```python
from build123d import *
from OCP.BRepFilletAPI import BRepFilletAPI_MakeChamfer

# Parameters (mm, degrees)
SKETCH_1_W               = 70
SKETCH_1_H               = 60
EXTRUDE_1_DEPTH          = 15
SKETCH_2_R               = 11.5
EXTRUDE_3_DEPTH          = 5
CUT_EXTRUDE_1_DEPTH      = 69.745908969
CUT_EXTRUDE_1_DEPTH_BACK = 69.745908969
SKETCH_3_W               = 50
SKETCH_3_H               = 5
CHAMFER_1_SIZE           = 1.2
CHAMFER_1_SIZE2          = 0.692820323
CHAMFER_2_SIZE           = 1.2
CHAMFER_2_SIZE_2         = 0.692820323
CHAMFER_3_SIZE           = 1.2
CHAMFER_3_SIZE_2         = 0.692820323
CHAMFER_4_SIZE           = 1.2
CHAMFER_4_SIZE2          = 0.692820323


with BuildPart() as part:
    # 스케치1 → 보스-돌출1 (new body)
    with BuildSketch(Plane(origin=(0, 0, 0), x_dir=(1, 0, 0), z_dir=(0, 1, 0))):
        Rectangle(SKETCH_1_W, SKETCH_1_H)
    extrude(amount=EXTRUDE_1_DEPTH)

    # 스케치2 → 보스-돌출3 (add, symmetric)
    with BuildSketch(Plane(origin=(0, 0, 0), x_dir=(0, 0, -1), z_dir=(1, 0, 0))):
        with BuildLine():
            ThreePointArc((30, 15), (21.27501926, 22.183346174), (18, 33))
            ThreePointArc((18, 33), (0, 51), (-18, 33))
            ThreePointArc((-18, 33), (-21.27501926, 22.183346174), (-30, 15))
            Line((-30, 15), (30, 15))
        make_face()
        with Locations((0, 33)):
            Circle(SKETCH_2_R, mode=Mode.SUBTRACT)
    extrude(amount=EXTRUDE_3_DEPTH, both=True)

    # 스케치3 → 컷-돌출1 (cut, two sides: drawn at the far end of the back side and taken through both)
    with BuildSketch(Plane(origin=(0, 0, 0), x_dir=(0, 0, -1), z_dir=(1, 0, 0)).offset(-CUT_EXTRUDE_1_DEPTH_BACK)):
        with Locations((0, 7.5)):
            Rectangle(SKETCH_3_W, SKETCH_3_H)
    extrude(amount=CUT_EXTRUDE_1_DEPTH + CUT_EXTRUDE_1_DEPTH_BACK, mode=Mode.SUBTRACT)

    # 모따기1: one chamfer whose edges measure the first distance from different faces: ONE call of the kernel's chamfer builder (chamfer() names one face for all edges)
    chamfer_1_edges_1 = [part.edges().sort_by_distance(p)[0] for p in [
        (0, 0, 30),
    ]]
    chamfer_1_side_1 = [part.faces().sort_by_distance(p)[0] for p in [
        (0, 7.5, 30),
    ]]
    chamfer_1_edges_2 = [part.edges().sort_by_distance(p)[0] for p in [
        (-35, 0, 0),
    ]]
    chamfer_1_side_2 = [part.faces().sort_by_distance(p)[0] for p in [
        (-35, 7.5, -29.381534156),
    ]]
    chamfer_1_edges_3 = [part.edges().sort_by_distance(p)[0] for p in [
        (0, 0, -30),
    ]]
    chamfer_1_side_3 = [part.faces().sort_by_distance(p)[0] for p in [
        (0, 7.5, -30),
    ]]
    chamfer_1_edges_4 = [part.edges().sort_by_distance(p)[0] for p in [
        (35, 0, 0),
    ]]
    chamfer_1_side_4 = [part.faces().sort_by_distance(p)[0] for p in [
        (35, 7.5, 29.381534156),
    ]]
    chamfer_1 = BRepFilletAPI_MakeChamfer(part.part.solid().wrapped)
    for e in chamfer_1_edges_1:
        chamfer_1.Add(CHAMFER_1_SIZE, CHAMFER_1_SIZE2, e.wrapped, chamfer_1_side_1[0].wrapped)  # the first distance lies on this face
    for e in chamfer_1_edges_2:
        chamfer_1.Add(CHAMFER_1_SIZE, CHAMFER_1_SIZE2, e.wrapped, chamfer_1_side_2[0].wrapped)  # the first distance lies on this face
    for e in chamfer_1_edges_3:
        chamfer_1.Add(CHAMFER_1_SIZE, CHAMFER_1_SIZE2, e.wrapped, chamfer_1_side_3[0].wrapped)  # the first distance lies on this face
    for e in chamfer_1_edges_4:
        chamfer_1.Add(CHAMFER_1_SIZE, CHAMFER_1_SIZE2, e.wrapped, chamfer_1_side_4[0].wrapped)  # the first distance lies on this face
    add(Compound.cast(chamfer_1.Shape()), mode=Mode.REPLACE)

    # 모따기2
    # the kernel refuses this chamfer: 1.2, 0.98830445, 0.692820323 mm, written as the material it takes off along each edge
    with BuildSketch(Plane(origin=(-35, 15, -33.104502906), x_dir=(0, -1, 0), z_dir=(0, 0, 1)), Plane(origin=(35, 15, 33.104502906), x_dir=(0, -1, 0), z_dir=(0, 0, -1))) as chamfer_2_piece_1:
        Polygon((CHAMFER_2_SIZE, 0), (0, CHAMFER_2_SIZE_2), (0, 0), align=None)
    extrude(amount=66.209005811, mode=Mode.SUBTRACT)
    with BuildSketch(Plane(origin=(-5, 15, -30), x_dir=(0, 0, 1), z_dir=(-1, 0, 0)), Plane(origin=(38.104502906, 15, -30), x_dir=(0, 0, 1), z_dir=(-1, 0, 0))) as chamfer_2_piece_2:
        Polygon((CHAMFER_2_SIZE_2, 0), (0, -CHAMFER_2_SIZE), (0, 0), align=None)
    extrude(amount=33.104502906, mode=Mode.SUBTRACT)
    with BuildSketch(Plane(origin=(5, 15, 30), x_dir=(0, -1, 0), z_dir=(1, 0, 0)), Plane(origin=(-38.104502906, 15, 30), x_dir=(0, -1, 0), z_dir=(1, 0, 0))) as chamfer_2_piece_3:
        Polygon((CHAMFER_2_SIZE, 0), (0, CHAMFER_2_SIZE_2), (0, 0), align=None)
    extrude(amount=33.104502906, mode=Mode.SUBTRACT)
    with BuildSketch(Plane(origin=(-5, 15, -30), x_dir=(0, -1, 0), z_dir=(1, 0, 0)), Plane(origin=(5, 15, 30), x_dir=(0, -1, 0), z_dir=(-1, 0, 0))) as chamfer_2_piece_4:
        with BuildLine():
            Line((CHAMFER_2_SIZE, 0), (-0.41845847, -0.934417434))
            ThreePointArc((-0.41845847, -0.934417434), (-0.211061153, -0.487718993), (0, 0))
            Line((0, 0), (CHAMFER_2_SIZE, 0))
        make_face()
    extrude(amount=10, mode=Mode.SUBTRACT)

    # 모따기3
    # the kernel refuses this chamfer: 1.2, 0.692820323 mm, written as the material it takes off along each edge
    with BuildSketch(Plane(origin=(5, 33, -37.5), x_dir=(0, -0.958795780822353, 0.2840961996881595), z_dir=(0, -0.2840961996881595, -0.958795780822353))) as chamfer_3_piece_1_section:
        Polygon((19.5 + CHAMFER_3_SIZE, 0), (19.5, CHAMFER_3_SIZE_2), (19.5, 0), align=None)
    chamfer_3_piece_1 = revolve(axis=Axis((5, 33, -37.5), (-1, 0, 0)), revolution_arc=73.495168323, mode=Mode.PRIVATE)
    chamfer_3_piece_1 = split(chamfer_3_piece_1, bisect_by=Plane(origin=(5, 15, -37.5), z_dir=(0, 1, 0)), keep=Keep.TOP, mode=Mode.PRIVATE)
    add(chamfer_3_piece_1, mode=Mode.SUBTRACT)
    with BuildSketch(Plane(origin=(5, 33, 37.5), x_dir=(0, 0, -1), z_dir=(0, 1, 0))) as chamfer_3_piece_2_section:
        Polygon((19.5, CHAMFER_3_SIZE_2), (19.5 + CHAMFER_3_SIZE, 0), (19.5, 0), align=None)
    chamfer_3_piece_2 = revolve(axis=Axis((5, 33, 37.5), (-1, 0, 0)), revolution_arc=73.495168323, mode=Mode.PRIVATE)
    chamfer_3_piece_2 = split(chamfer_3_piece_2, bisect_by=Plane(origin=(5, 15, 37.5), z_dir=(0, 1, 0)), keep=Keep.TOP, mode=Mode.PRIVATE)
    add(chamfer_3_piece_2, mode=Mode.SUBTRACT)
    with BuildSketch(Plane(origin=(5, 33, 0), x_dir=(0, 0, -1), z_dir=(0, -1, 0))) as chamfer_3_piece_3:
        Polygon((18 - CHAMFER_3_SIZE, 0), (18, -CHAMFER_3_SIZE_2), (18, 0), align=None)
    revolve(axis=Axis((5, 33, 0), (1, 0, 0)), revolution_arc=180, mode=Mode.SUBTRACT)
    with BuildSketch(Plane(origin=(-5, 33, -37.5), x_dir=(0, -0.958795780822353, 0.2840961996881595), z_dir=(0, -0.2840961996881595, -0.958795780822353))) as chamfer_3_piece_4_section:
        Polygon((19.5 + CHAMFER_3_SIZE, 0), (19.5, -CHAMFER_3_SIZE_2), (19.5, 0), align=None)
    chamfer_3_piece_4 = revolve(axis=Axis((-5, 33, -37.5), (-1, 0, 0)), revolution_arc=73.495168323, mode=Mode.PRIVATE)
    chamfer_3_piece_4 = split(chamfer_3_piece_4, bisect_by=Plane(origin=(-5, 15, -37.5), z_dir=(0, 1, 0)), keep=Keep.TOP, mode=Mode.PRIVATE)
    add(chamfer_3_piece_4, mode=Mode.SUBTRACT)
    with BuildSketch(Plane(origin=(-5, 33, 0), x_dir=(0, 0, -1), z_dir=(0, -1, 0))) as chamfer_3_piece_5:
        Polygon((18 - CHAMFER_3_SIZE, 0), (18, CHAMFER_3_SIZE_2), (18, 0), align=None)
    revolve(axis=Axis((-5, 33, 0), (1, 0, 0)), revolution_arc=180, mode=Mode.SUBTRACT)
    with BuildSketch(Plane(origin=(-5, 33, 37.5), x_dir=(0, 0, -1), z_dir=(0, 1, 0))) as chamfer_3_piece_6_section:
        Polygon((19.5, -CHAMFER_3_SIZE_2), (19.5 + CHAMFER_3_SIZE, 0), (19.5, 0), align=None)
    chamfer_3_piece_6 = revolve(axis=Axis((-5, 33, 37.5), (-1, 0, 0)), revolution_arc=73.495168323, mode=Mode.PRIVATE)
    chamfer_3_piece_6 = split(chamfer_3_piece_6, bisect_by=Plane(origin=(-5, 15, 37.5), z_dir=(0, 1, 0)), keep=Keep.TOP, mode=Mode.PRIVATE)
    add(chamfer_3_piece_6, mode=Mode.SUBTRACT)

    # 모따기4: one chamfer whose edges measure the first distance from different faces: ONE call of the kernel's chamfer builder (chamfer() names one face for all edges)
    chamfer_4_edges_1 = [part.edges().sort_by_distance(p)[0] for p in [
        (-35, 7.5, 25),
    ]]
    chamfer_4_side_1 = [part.faces().sort_by_distance(p)[0] for p in [
        (0, 7.5, 25),
    ]]
    chamfer_4_edges_2 = [part.edges().sort_by_distance(p)[0] for p in [
        (-35, 10, 0),
    ]]
    chamfer_4_side_2 = [part.faces().sort_by_distance(p)[0] for p in [
        (0, 10, 0),
    ]]
    chamfer_4_edges_3 = [part.edges().sort_by_distance(p)[0] for p in [
        (-35, 7.5, -25),
    ]]
    chamfer_4_side_3 = [part.faces().sort_by_distance(p)[0] for p in [
        (0, 7.5, -25),
    ]]
    chamfer_4_edges_4 = [part.edges().sort_by_distance(p)[0] for p in [
        (-35, 5, 0),
    ]]
    chamfer_4_side_4 = [part.faces().sort_by_distance(p)[0] for p in [
        (0, 5, 0),
    ]]
    chamfer_4_edges_5 = [part.edges().sort_by_distance(p)[0] for p in [
        (35, 7.5, 25),
        (35, 5, 0),
        (35, 7.5, -25),
        (35, 10, 0),
    ]]
    chamfer_4_side_5 = [part.faces().sort_by_distance(p)[0] for p in [
        (35, 1.813087269, 0),
    ]]
    chamfer_4 = BRepFilletAPI_MakeChamfer(part.part.solid().wrapped)
    for e in chamfer_4_edges_1:
        chamfer_4.Add(CHAMFER_4_SIZE, CHAMFER_4_SIZE2, e.wrapped, chamfer_4_side_1[0].wrapped)  # the first distance lies on this face
    for e in chamfer_4_edges_2:
        chamfer_4.Add(CHAMFER_4_SIZE, CHAMFER_4_SIZE2, e.wrapped, chamfer_4_side_2[0].wrapped)  # the first distance lies on this face
    for e in chamfer_4_edges_3:
        chamfer_4.Add(CHAMFER_4_SIZE, CHAMFER_4_SIZE2, e.wrapped, chamfer_4_side_3[0].wrapped)  # the first distance lies on this face
    for e in chamfer_4_edges_4:
        chamfer_4.Add(CHAMFER_4_SIZE, CHAMFER_4_SIZE2, e.wrapped, chamfer_4_side_4[0].wrapped)  # the first distance lies on this face
    for e in chamfer_4_edges_5:
        chamfer_4.Add(CHAMFER_4_SIZE, CHAMFER_4_SIZE2, e.wrapped, chamfer_4_side_5[0].wrapped)  # the first distance lies on this face
    add(Compound.cast(chamfer_4.Shape()), mode=Mode.REPLACE)


solid = part.part
```
Geometry check sheet. Reference: the model listing, model coordinates, mm. A direction names the side the tool comes from. Coordinates: 2 decimals unless noted, no trailing zeros. Order: outer loops, then holes, each group sorted by start corner. A loop starts at its lowest first (then second) coordinate and runs counter-clockwise, first axis right, second up. Notation, with made-up numbers: (60.5, 22) - (103.5, 22) arc R12 cw to (103.5, 28) - close; hole circle Ø2 at (51, -27.5). An arc over 180 degrees is marked (long way). Answer as a JSON object with one key per item and string values. Group by question number.
Item 1: Scan lines: probe 1 along Y at (x, z) = (-1.75, 0); probe 2 along Y at (x, z) = (-28, -13.5); probe 3 along X at (y, z) = (23.5, -8.5). Record each from-to range of solid material in increasing order.
Item 2: Sectioned sample at B-B, the plane x = -1.5. Record the cut outline in (y, z), and give its area (3 significant figures).
Item 3: Sectioned sample at C-C, the plane x = 19.5. Record the cut outline in (y, z).
Item 4: Depth check by flat-ended pin: pin 1 Ø18.5 at (y, z) = (33, 0) entering from -X; pin 2 Ø5 at (y, z) = (22, 15.5) entering from -X; pin 3 Ø12 at (y, z) = (21.5, -14.5) entering from +X; pin 4 Ø9 at (x, z) = (-17, -10) entering from +Y. Enter the tip coordinate at first touch or a pass-through.
Item 5: Tool access check on faces 4 (the face through (5, 21, 0)), 5 (the face through (0, 5, 0)), 6 (the face through (-5, 21, 0)). Record the directions out of +Z, -Z, +X, -X, +Y, -Y that give a thin tool (end or side, any length) a straight path to the whole face; none if there is none.
Item 6: Draft check along Y on faces 1 (the face through (0, 7, 30)), 2 (the face through (-0.07, 21.773, 2.493)), 3 (the face through (-20, 15, 0)). Enter one of: +Y half, -Y half, draft (parallel to the pull), parting line (faces both ways), or undercut.
Item 7: Sectioned sample at A-A, the plane z = 0. Record the cut outline in (x, y), and give its area (3 significant figures).
Resolved:
{
 "1": {"probe 1": "0 to 5, 10 to 21.5, 44.5 to 51", "probe 2": "0 to 5, 10 to 15", "probe 3": "-5 to 5"},
 "2": {"outline": "(0, -29.31) - (1.2, -30) - (13.8, -30) - (15.42, -29.07) arc R19.5 cw to (33, -18) arc R18 ccw to (33, 18) arc R19.5 cw to (15.42, 29.07) - (13.8, 30) - (1.2, 30) - (0, 29.31) - close; hole (5, -25) - (10, -25) - (10, 25) - (5, 25) - close; hole circle Ø23 at (33, 0)", "area": "1,510 mm^2"},
 "3": {"outline": "(0, -29.31) - (1.2, -30) - (13.8, -30) - (15, -29.31) - (15, 29.31) - (13.8, 30) - (1.2, 30) - (0, 29.31) - close; hole (5, -25) - (10, -25) - (10, 25) - (5, 25) - close"},
 "4": {"pin 1": "through", "pin 2": "x = -5", "pin 3": "x = 5", "pin 4": "y = 15"},
 "5": {"face 4": "+Z, -Z, +X, +Y", "face 5": "+X, -X", "face 6": "+Z, -Z, -X, +Y"},
 "6": {"face 1": "draft", "face 2": "undercut", "face 3": "+Y half"},
 "7": {"outline": "(-35, 1.2) - (-34.31, 0) - (34.31, 0) - (35, 1.2) - (35, 3.8) - (34.31, 5) - (-33.8, 5) - (-35, 4.31) - close; (-35, 10.69) - (-33.8, 10) - (34.31, 10) - (35, 11.2) - (35, 13.8) - (34.31, 15) - (5, 15) - (5, 21.5) - (-5, 21.5) - (-5, 15) - (-34.31, 15) - (-35, 13.8) - close; (-5, 44.5) - (5, 44.5) - (5, 49.8) - (4.31, 51) - (-4.31, 51) - (-5, 49.8) - close", "area": "826 mm^2"}
}
